from build123d import *

# Parameters (mm, degrees)
SKETCH1_R           = 1.7526
BOSS_EXTRUDE1_DEPTH = 3.175
FILLET1_R           = 5.08
FILLET2_R           = 5.08
SKETCH2_R           = 2.0828
SKETCH2_R_2         = 7.9375
CUT_EXTRUDE1_DEPTH  = 49.775275499


with BuildPart() as part:
    # Sketch1 → Boss-Extrude1 (new, symmetric)
    with BuildSketch(Plane(origin=(0, 0, 0), x_dir=(1, 0, 0), z_dir=(0, 1, 0))):
        Polygon((-19.05, -38.1), (-6.35, -38.1), (-6.35, -44.45), (6.35, -44.45), (6.35, -38.1), (19.05, -38.1), (19.05, -29.9466), (9.525, 0), (-9.525, 0), (-19.05, -29.9466), align=None)
        with Locations(Location((0, -41.275, 0), (0, 0, 270))):
            Circle(SKETCH1_R, mode=Mode.SUBTRACT)
    extrude(amount=BOSS_EXTRUDE1_DEPTH, both=True)

    # Fillet1
    fillet1_edges = [part.edges().sort_by_distance(p)[0] for p in [
        (-9.525, 0, 0),
        (9.525, 0, 0),
    ]]
    fillet(fillet1_edges, radius=FILLET1_R)

    # Fillet2
    fillet2_edges = [part.edges().sort_by_distance(p)[0] for p in [
        (-19.05, 0, 29.9466),
        (19.05, 0, 29.9466),
    ]]
    fillet(fillet2_edges, radius=FILLET2_R)

    # Sketch2 → Cut-Extrude1 (cut, through all)
    with BuildSketch(Plane(origin=(0, 3.175, 0), x_dir=(1, 0, 0), z_dir=(0, 1, 0))):
        with Locations(Location((0, -7.14375, 0), (0, 0, 270))):
            Circle(SKETCH2_R)
        with Locations(Location((0, -19.05, 0), (0, 0, 270))):
            Circle(SKETCH2_R_2)
        with Locations(Location((0, -30.95625, 0), (0, 0, 90))):
            Circle(SKETCH2_R)
    extrude(amount=-CUT_EXTRUDE1_DEPTH, mode=Mode.SUBTRACT)


solid = part.part
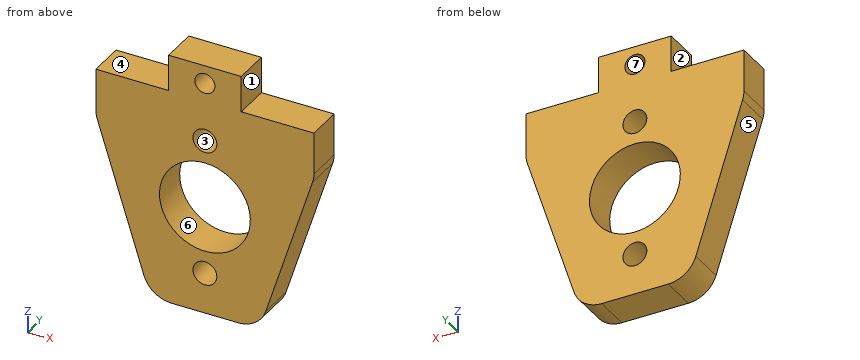
Read the model definition and answer for the solid it produces. Units are mm, in the model's axes. Face numbers are marked on the shaded views. A direction names the side the tool comes from. Round coordinates to 2 decimals unless told otherwise and drop trailing zeros. Loops run counter-clockwise (first coordinate to the right, second up) from the corner with the lowest first, then second, coordinate; pieces in that order, holes last. Notation, with made-up numbers: (85, 20) - (99, 20) arc R20 cw to (99, 30) - close; hole circle Ø8 at (48, 27.5). An arc over 180 degrees is marked (long way). One line per question, with ' | ' between items. Start each with the question number.
Q1. Section D-D on x = -8.5 is taken. Give the vertices of the cut face in (y, z) (3 decimals).
Q2. Find the intervals of material crossed by L1, parallel to Z at x = 1.5, y = 2.5; L2, parallel to X at y = -0.75, z = 19.05; L3, parallel to Z at x = 2.5, y = 2.25, in increasing order.
Q3. Section A-A on x = 0 is taken. Count the separate pieces of the cut face and the enclosed holes in it, plus the area to 3 significant figures.
Q4. For a pull along Z with two mould halves and no side action, classify the marked faces 4, 5, 6 and 7 as +Z half, -Z half, draft (parallel to the pull), parting line (faces both ways), or undercut.
Q5. For the marked faces 1, 2 and 3, determine the directions among +Z, -Z, +X, -X, +Y, -Y from which every point of the face is accessible in a straight line to the end or side of a thin tool.
Q6. Flat-ended cylindrical pins translate along their axes: pin 1 (3 mm diameter, centred on x = 13.5, y = 0.5, fed in from +Z); pin 2 (2 mm diameter, centred on y = 2.5, z = 29, fed in from -X). Find the tip coordinate at first contact, or state that the pin passes through.
Q7. Section C-C on z = 19.05 is taken. Give the vertices of the cut face in (x, y) (1 decimal).
Established:
1) outline: (-3.175, 0.771) - (3.175, 0.771) - (3.175, 38.1) - (-3.175, 38.1) - close
2) L1: 0 to 5.7, 8.59 to 11.26, 26.84 to 29.51, 32.4 to 40.37, 42.18 to 44.45 | L2: -15.58 to -7.94, 7.94 to 15.58 | L3: 0 to 11.52, 26.58 to 44.45
3) separate pieces: 5 | enclosed holes: 0 | area: 106 mm²
4) face 4: +Z half | face 5: -Z half | face 6: undercut | face 7: undercut
5) face 1: +Z, +X, +Y, -Y | face 2: +Z, -X, +Y, -Y | face 3: +Y, -Y
6) pin 1: z = 38.1 | pin 2: x = -19
7) outline: (-15.6, -3.2) - (-7.9, -3.2) - (-7.9, 3.2) - (-15.6, 3.2) - close; (7.9, -3.2) - (15.6, -3.2) - (15.6, 3.2) - (7.9, 3.2) - close
